Part model, mm, in its own coordinate system. A direction names the side the tool comes from. Round coordinates to 2 decimals unless told otherwise and drop trailing zeros. Answer as a JSON object with one key per item and string values. Group by question number.
```python
from build123d import *

# Parameters (mm, degrees)
POCKET_DEPTH = 1.25


with BuildPart() as part:
    # Sketch (on DatumPlane) → Revolution (revolve)
    with BuildSketch(Plane.YZ):
        Polygon((0, 0), (0, -2.5), (19.75, -2.5), (20, -2.25), (20, -0.25), (19.75, 0), align=None)
    revolve(axis=Axis((0, 0, 0), (0, 0, 1)))

    # Sketch005 → Pocket (cut)
    with BuildSketch(Plane.XY):
        with BuildLine():
            add(Edge.make_bspline(
                [(-3.689668, 13.94616), (-2.641611, 15.462794), (-1.516137, 17.02899), (0.085841, 18)],
                knots=[0, 0, 0, 0, 1, 1, 1, 1], degree=3))
            add(Edge.make_bspline(
                [(0.085841, 18), (1.66552, 17.053067), (2.779956, 15.514726), (3.813048, 14.024985)],
                knots=[0, 0, 0, 0, 1, 1, 1, 1], degree=3))
            add(Edge.make_bspline(
                [(3.813048, 14.024985), (6.246463, 10.339042), (7.734204, 5.911748), (7.434093, 1.462081)],
                knots=[0, 0, 0, 0, 1, 1, 1, 1], degree=3))
            add(Edge.make_bspline(
                [(7.434093, 1.462081), (8.220487, 0.802888), (9.029626, 0.169994), (9.804315, -0.502683)],
                knots=[0, 0, 0, 0, 1, 1, 1, 1], degree=3))
            add(Edge.make_bspline(
                [(9.804315, -0.502683), (10.91638, -1.524811), (11.43563, -3.119232), (11.167893, -4.601492)],
                knots=[0, 0, 0, 0, 1, 1, 1, 1], degree=3))
            add(Edge.make_bspline(
                [(11.167893, -4.601492), (10.794809, -6.473948), (10.436246, -8.350627), (10.041382, -10.217971)],
                knots=[0, 0, 0, 0, 1, 1, 1, 1], degree=3))
            add(Edge.make_bspline(
                [(10.041382, -10.217971), (9.821873, -11.178684), (8.522081, -11.618517), (7.757911, -11.004736)],
                knots=[0, 0, 0, 0, 1, 1, 1, 1], degree=3))
            add(Edge.make_bspline(
                [(7.757911, -11.004736), (6.48953, -9.946011), (5.252709, -8.848319), (3.984699, -7.78826)],
                knots=[0, 0, 0, 0, 1, 1, 1, 1], degree=3))
            add(Edge.make_bspline(
                [(3.984699, -7.78826), (3.02532, -8.711487), (1.750864, -9.327119), (0.412845, -9.401277)],
                knots=[0, 0, 0, 0, 1, 1, 1, 1], degree=3))
            add(Edge.make_bspline(
                [(0.412845, -9.401277), (-1.127422, -9.509883), (-2.652353, -8.871136), (-3.769011, -7.827598)],
                knots=[0, 0, 0, 0, 1, 1, 1, 1], degree=3))
            add(Edge.make_bspline(
                [(-3.769011, -7.827598), (-4.678754, -8.524056), (-5.522267, -9.360086), (-6.411119, -10.106031)],
                knots=[0, 0, 0, 0, 1, 1, 1, 1], degree=3))
            add(Edge.make_bspline(
                [(-6.411119, -10.106031), (-6.840728, -10.45126), (-7.197958, -10.904946), (-7.706392, -11.140679)],
                knots=[0, 0, 0, 0, 1, 1, 1, 1], degree=3))
            add(Edge.make_bspline(
                [(-7.706392, -11.140679), (-8.494639, -11.47887), (-9.509729, -10.97414), (-9.687899, -10.126849)],
                knots=[0, 0, 0, 0, 1, 1, 1, 1], degree=3))
            add(Edge.make_bspline(
                [(-9.687899, -10.126849), (-10.093802, -8.301287), (-10.517855, -6.478985), (-10.911756, -4.650609)],
                knots=[0, 0, 0, 0, 1, 1, 1, 1], degree=3))
            add(Edge.make_bspline(
                [(-10.911756, -4.650609), (-11.23187, -3.103897), (-10.66491, -1.419835), (-9.473131, -0.38289)],
                knots=[0, 0, 0, 0, 1, 1, 1, 1], degree=3))
            add(Edge.make_bspline(
                [(-9.473131, -0.38289), (-8.783193, 0.19659), (-8.083624, 0.764438), (-7.380796, 1.328138)],
                knots=[0, 0, 0, 0, 1, 1, 1, 1], degree=3))
            add(Edge.make_bspline(
                [(-7.380796, 1.328138), (-7.184994, 1.431114), (-7.283376, 1.668625), (-7.272264, 1.843092)],
                knots=[0, 0, 0, 0, 1, 1, 1, 1], degree=3))
            add(Edge.make_bspline(
                [(-7.272264, 1.843092), (-7.481771, 6.136295), (-6.015292, 10.379862), (-3.689668, 13.94616)],
                knots=[0, 0, 0, 0, 1, 1, 1, 1], degree=3))
        make_face()
        with BuildLine():
            add(Edge.make_bspline(
                [(-2.444846, 8.291231), (-3.365257, 7.106342), (-3.25391, 5.271002), (-2.186443, 4.212795)],
                knots=[0, 0, 0, 0, 1, 1, 1, 1], degree=3))
            add(Edge.make_bspline(
                [(-2.186443, 4.212795), (-1.056302, 2.967529), (1.084336, 2.922115), (2.26641, 4.117228)],
                knots=[0, 0, 0, 0, 1, 1, 1, 1], degree=3))
            add(Edge.make_bspline(
                [(2.26641, 4.117228), (3.178894, 4.950888), (3.487451, 6.350544), (3.051916, 7.500688)],
                knots=[0, 0, 0, 0, 1, 1, 1, 1], degree=3))
            add(Edge.make_bspline(
                [(3.051916, 7.500688), (2.652829, 8.609493), (1.584399, 9.441301), (0.409289, 9.544721)],
                knots=[0, 0, 0, 0, 1, 1, 1, 1], degree=3))
            add(Edge.make_bspline(
                [(0.409289, 9.544721), (-0.675884, 9.669626), (-1.799506, 9.170378), (-2.444846, 8.291231)],
                knots=[0, 0, 0, 0, 1, 1, 1, 1], degree=3))
        make_face(mode=Mode.SUBTRACT)
        with BuildLine():
            add(Edge.make_bspline(
                [(-4.128908, -11.658892), (-4.144688, -11.120603), (-3.474752, -10.750482), (-3.021955, -11.035333)],
                knots=[0, 0, 0, 0, 1, 1, 1, 1], degree=3))
            add(Edge.make_bspline(
                [(-3.021955, -11.035333), (-1.105419, -12.022123), (1.276879, -12.021678), (3.193341, -11.034814)],
                knots=[0, 0, 0, 0, 1, 1, 1, 1], degree=3))
            add(Edge.make_bspline(
                [(3.193341, -11.034814), (3.633173, -10.76478), (4.285033, -11.089117), (4.301257, -11.612886)],
                knots=[0, 0, 0, 0, 1, 1, 1, 1], degree=3))
            add(Edge.make_bspline(
                [(4.301257, -11.612886), (4.307702, -12.75614), (4.309036, -13.90058), (4.303035, -15.044204)],
                knots=[0, 0, 0, 0, 1, 1, 1, 1], degree=3))
            add(Edge.make_bspline(
                [(4.303035, -15.044204), (4.311851, -15.602274), (3.574648, -15.95817), (3.141334, -15.609164)],
                knots=[0, 0, 0, 0, 1, 1, 1, 1], degree=3))
            add(Edge.make_bspline(
                [(3.141334, -15.609164), (2.811515, -15.318312), (2.514071, -14.991235), (2.196772, -14.686011)],
                knots=[0, 0, 0, 0, 1, 1, 1, 1], degree=3))
            add(Edge.make_bspline(
                [(2.196772, -14.686011), (1.694783, -15.663985), (1.221613, -16.656776), (0.715475, -17.632454)],
                knots=[0, 0, 0, 0, 1, 1, 1, 1], degree=3))
            add(Edge.make_bspline(
                [(0.715475, -17.632454), (0.472408, -18.097326), (-0.287094, -18.100512), (-0.534829, -17.640232)],
                knots=[0, 0, 0, 0, 1, 1, 1, 1], degree=3))
            add(Edge.make_bspline(
                [(-0.534829, -17.640232), (-1.043782, -16.662703), (-1.513692, -15.663985), (-2.02546, -14.687419)],
                knots=[0, 0, 0, 0, 1, 1, 1, 1], degree=3))
            add(Edge.make_bspline(
                [(-2.02546, -14.687419), (-2.338166, -14.995383), (-2.636499, -15.320683), (-2.965874, -15.61109)],
                knots=[0, 0, 0, 0, 1, 1, 1, 1], degree=3))
            add(Edge.make_bspline(
                [(-2.965874, -15.61109), (-3.397335, -15.9618), (-4.133131, -15.599088), (-4.12713, -15.044575)],
                knots=[0, 0, 0, 0, 1, 1, 1, 1], degree=3))
            add(Edge.make_bspline(
                [(-4.12713, -15.044575), (-4.136316, -13.916359), (-4.130315, -12.787626), (-4.128908, -11.658892)],
                knots=[0, 0, 0, 0, 1, 1, 1, 1], degree=3))
        make_face()
        with BuildLine():
            add(Edge.make_bspline(
                [(1.60366, 6.366324), (1.60366, 9.036838), (-0.709074, 7.701581), (-3.021807, 6.366324), (-0.709074, 5.031066), (1.60366, 3.695809), (1.60366, 6.366324)],
                knots=[0, 0, 0, 2.094395, 2.094395, 4.18879, 4.18879, 6.283185, 6.283185, 6.283185], degree=2, weights=[1, 0.5, 1, 0.5, 1, 0.5, 1]))
        make_face()
    extrude(amount=-POCKET_DEPTH, mode=Mode.SUBTRACT)


solid = part.part
```
Q1. Two-plate mould, pull along X, no slides. Class faces 1 (the cylindrical face through (19.524, -4.336, -1.236)), 2 (the flat face through (0, 0, -2.5)), 3 (the flat face through (0, 0, -1.25)): +X half, -X half, draft (parallel to the pull), parting line (faces both ways), or undercut.
Q2. Band-saw the part on A-A (z = -0.7). Count the separate pieces of the cut face and the enclosed holes in it, plus the area to 3 significant figures.
Q3. Which spindle directions (+Z, -Z, +X, -X, +Y, -Y) get a long thin tool onto all of the face, cutting with end or side? Do faces 4 (the flat face through (1, 8, 0)), 5 (the flat face through (0, 7, -1.25)). Say none if no direction does.
Q4. Wall check: line 1 (Y direction, x = -0.5, z = -0.15); line 2 (X direction, y = -8.5, z = -0.9); line 3 (Z direction, x = 1, y = 3). Give the ranges that are in metal, low to high. Write a range as [from, to].
Completed:
{
 "1": {"face 1": "parting line", "face 2": "draft", "face 3": "undercut"},
 "2": {"separate pieces": "2", "enclosed holes": "3", "area": "840 mm2"},
 "3": {"face 4": "+Z, +X, -X, +Y, -Y", "face 5": "+Z"},
 "4": {"line 1": "[-19.89, -17.7], [-11.75, -9.38], [3.3, 4.93], [7.8, 9.51], [17.6, 19.89]", "line 2": "[-18.1, -10.05], [-4.59, -2.91], [3.09, 4.83], [10.4, 18.1]", "line 3": "[-2.5, -1.25]"}
}
